Check sheet for the modelled part. Datum: model origin and axes. Units: mm. A direction names the side the tool comes from. Give positions to 0.01 mm unless a question says otherwise; leave off trailing zeros. Order: outer loops, then holes, each group sorted by start corner. A loop starts at its lowest first (then second) coordinate and runs counter-clockwise, first axis right, second up.
```python
from build123d import *

# Parameters (mm, degrees)
BOSS_EXTRUDE1_DEPTH = 63.5
SKETCH3_R           = 1.5875
CUT_EXTRUDE1_DEPTH  = 63.5


with BuildPart() as part:
    # Sketch2 → Boss-Extrude1 (new body)
    with BuildSketch(Plane(origin=(0, 0, 0), x_dir=(1, 0, 0), z_dir=(0, 1, 0))):
        Polygon((16.764, 6.1722), (25.4, 6.1722), (25.4, 0), (0, 0), (0, 6.1722), (8.636, 6.1722), (8.636, 9.9822), (16.764, 9.9822), align=None)
    extrude(amount=BOSS_EXTRUDE1_DEPTH)

    # Sketch3 → Cut-Extrude1 (cut)
    with BuildSketch(Plane.XY):
        with Locations((12.7, 50.8)):
            Circle(SKETCH3_R)
        with Locations((12.7, 12.7)):
            Circle(SKETCH3_R)
    extrude(amount=-CUT_EXTRUDE1_DEPTH, mode=Mode.SUBTRACT)


solid = part.part
```
Q1. Go/stop test with flat-tipped pins: P1, Ø8, axis at x = 22.5, y = 45, coming from the -Z side; P2, Ø1.5, axis at y = 56, z = -7.5, coming from the +X side; P3, Ø1.9, axis at x = 12.7, y = 50.8, coming from the -Z side; P4, Ø4, axis at y = 43.5, z = -8.5, coming from the -X side. Record where each tip stops, or that it passes through.
Q2. Sectioned sample at B-B, the plane y = 50.8. Record the cut outline in (x, z).
Q3. Draft check along X on faces 1 (the flat face through (0, 31, -3)), 2 (the flat face through (4, 31, -6.172)), 3 (the flat face through (25.4, 31, -3)), 4 (the cylindrical face through (14.214, 13.177, -4.921)). Enter one of: pulls with the +X half, pulls with the -X half, needs draft (parallel to the pull), parting line crosses it, or undercut.
Q4. Sectioned sample at D-D, the plane y = 21.5. Record the cut outline in (x, z), plus the area to 3 significant figures.
Q5. Sectioned sample at C-C, the plane z = -7.5. Record the cut outline in (x, y) (1 decimal), plus the area to 3 significant figures.
Q6. Material ranges on line 1 (Y direction, x = 12.7, z = -4.5); line 2 (Y direction, x = 13.5, z = -0.25); line 3 (Z direction, x = 21, y = 7), recorded low to high.
Q7. Tool access check on faces 5 (the flat face through (13, 0, -4)), 6 (the flat face through (16.764, 31, -8)), 7 (the flat face through (8.636, 31, -8)). Record the directions out of +Z, -Z, +X, -X, +Y, -Y that give a thin tool (end or side, any length) a straight path to the whole face; none if there is none.
Q8. Sectioned sample at A-A, the plane x = 12.7. Record the cut outline in (y, z).
Filled in:
1. P1: stops at z = -6.17
1. P2: stops at x = 16.76
1. P3: passes through
1. P4: stops at x = 8.64
2. outline: (0, -6.17) - (8.64, -6.17) - (8.64, -9.98) - (11.11, -9.98) - (11.11, 0) - (0, 0) - close; (14.29, -9.98) - (16.76, -9.98) - (16.76, -6.17) - (25.4, -6.17) - (25.4, 0) - (14.29, 0) - close
3. face 1: pulls with the -X half
3. face 2: needs draft
3. face 3: pulls with the +X half
3. face 4: undercut
4. outline: (0, -6.17) - (8.64, -6.17) - (8.64, -9.98) - (16.76, -9.98) - (16.76, -6.17) - (25.4, -6.17) - (25.4, 0) - (0, 0) - close
4. area: 188 mm2
5. outline: (8.6, 0) - (16.8, 0) - (16.8, 63.5) - (8.6, 63.5) - close; hole circle Ø3.2 at (12.7, 12.7); hole circle Ø3.2 at (12.7, 50.8)
5. area: 500 mm2
6. line 1: y = 0 to 11.11, 14.29 to 49.21, 52.39 to 63.5
6. line 2: y = 0 to 11.33, 14.07 to 49.43, 52.17 to 63.5
6. line 3: z = -6.17 to 0
7. face 5: +Z, -Z, +X, -X, -Y
7. face 6: -Z, +X, +Y, -Y
7. face 7: -Z, -X, +Y, -Y
8. outline: (0, -9.98) - (11.11, -9.98) - (11.11, 0) - (0, 0) - close; (14.29, -9.98) - (49.21, -9.98) - (49.21, 0) - (14.29, 0) - close; (52.39, -9.98) - (63.5, -9.98) - (63.5, 0) - (52.39, 0) - close
